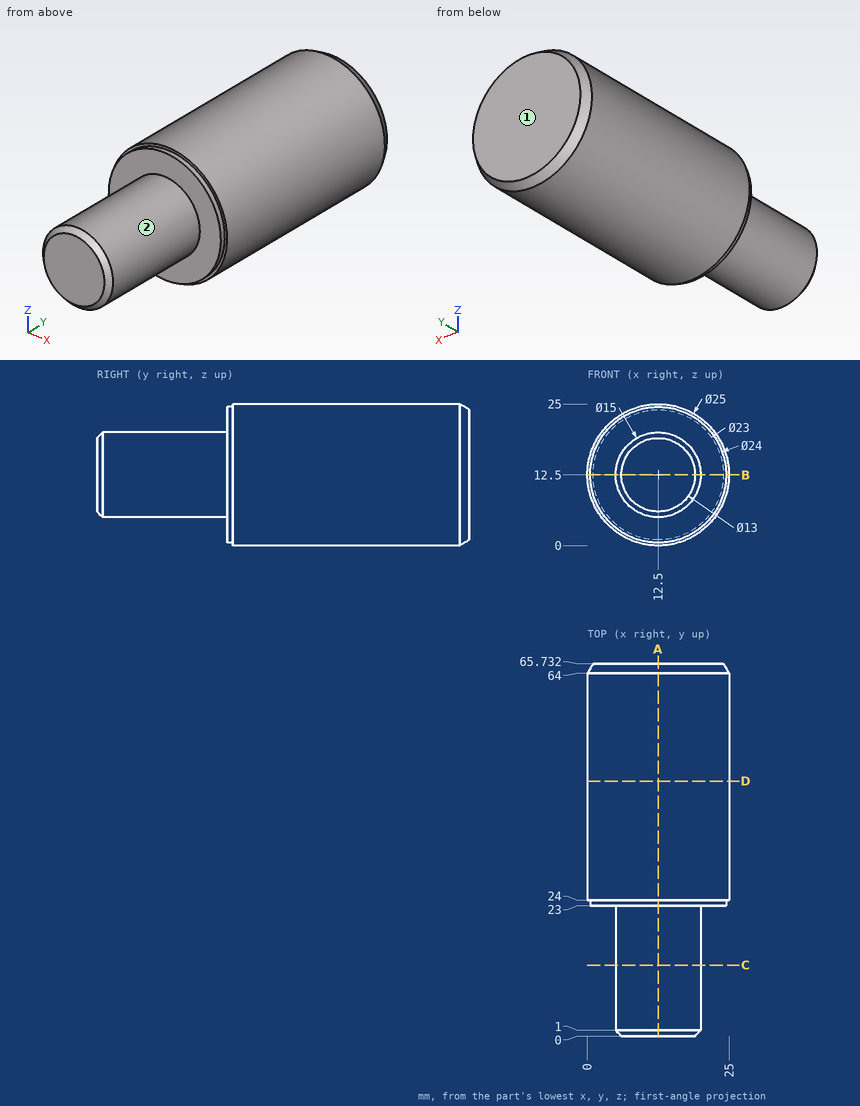
Geometry check sheet. Reference: drawing and pictorial views, mm from the part's lowest x, y, z. A direction names the side the tool comes from. Coordinates: 2 decimals unless noted, no trailing zeros. Write each loop counter-clockwise with the first axis right and the second up, starting at its lowest first coordinate (ties: lowest second). Pieces come first, ordered by that corner, then holes. Notation, with made-up numbers: (-40, 12.5) - (17, 12.5) arc R31 ccw to (17, 44.5) - close; hole circle Ø4 at (2, -18.75). An arc over 180 degrees is marked (long way). Write item = value, one per line.
Q1. Cross-section at C-C (y = 12.5). Enter the section's corners in (x, z).
Answer:
outline = circle Ø15 at (12.5, 12.5)
Q2. Cross-section at D-D (y = 45). Enter the section's corners in (x, z).
Answer:
outline = circle Ø25 at (12.5, 12.5)
Q3. Access from +Z, -Z, +X, -X, +Y, -Y to the whole of each face (thin tool, end or side, straight path). Record for the marked faces 1 and 2.
Answer:
face_1 = +Z, -Z, +X, -X, +Y
face_2 = -Y
Q4. Go/stop test with flat-tipped pins: pin 1 Ø7.5 at (x, z) = (18, 8) entering from -Y; pin 2 Ø3 at (y, z) = (32.5, 18.5) entering from +X; pin 3 Ø8 at (x, y) = (4.5, 37.5) entering from +Z; pin 4 Ø1 at (x, y) = (13, 9) entering from +Z. Record where each tip stops, or that it passes through.
Answer:
pin_1 = 0
pin_2 = 24.16
pin_3 = 24.34
pin_4 = 20
Q5. Cross-section at B-B (z = 12.5). Enter the section's corners in (x, y).
Answer:
outline = (0, 24) - (0.5, 24) - (0.5, 23) - (5, 23) - (5, 1) - (6, 0) - (19, 0) - (20, 1) - (20, 23) - (24.5, 23) - (24.5, 24) - (25, 24) - (25, 64) - (24, 65.73) - (1, 65.73) - (0, 64) - close
Q6. Material ranges on L1, parallel to Y at x = 21.5, z = 19.25; L2, parallel to Z at x = 18, y = 48 (3 decimals); L3, parallel to X at y = 60.5, z = 12.5, recorded low to high. Write a range as from..to.
Answer:
L1 = 23..65.73
L2 = 1.275..23.725
L3 = 0..25
Q7. Cross-section at A-A (x = 12.5). Enter the section's corners in (y, z), plus the area to 3 significant figures.
Answer:
outline = (0, 6) - (1, 5) - (23, 5) - (23, 0.5) - (24, 0.5) - (24, 0) - (64, 0) - (65.73, 1) - (65.73, 24) - (64, 25) - (24, 25) - (24, 24.5) - (23, 24.5) - (23, 20) - (1, 20) - (0, 19) - close
area = 1,410 mm²
